Verification items for the finished model (mm, model axes). A direction names the side the tool comes from. Coordinates: 2 decimals unless noted, no trailing zeros. Order: outer loops, then holes, each group sorted by start corner. A loop starts at its lowest first (then second) coordinate and runs counter-clockwise, first axis right, second up. Notation, with made-up numbers: M 87,48.5 L 108,48.5 A20 ccw 108,83.5 Z; hole C 38.25,62.5 d7. An arc over 180 degrees is marked long. Answer as a JSON object with one key per item and string values. Group by question number.
(1) Material ranges on line 1 (Y direction, x = 5.5, z = 5); line 2 (X direction, y = 0.5, z = 5.5); line 3 (X direction, y = -7.5, z = 2.25), recorded low to high.
(2) Cross-section at B-B (y = 2.5). Enter the section's corners in (x, z), plus the area to 3 significant figures.
(3) Cross-section at D-D (y = -5.5). Enter the section's corners in (x, z).
(4) Cross-section at C-C (x = 15). Enter the section's corners in (y, z), plus the area to 3 significant figures.
(5) Gauge pin test, flat end, axial feed: pin 1 Ø1.5 at (x, y) = (-1, 1) entering from -Z. Record the tip position at first contact, or that the pin passes through.
(6) Mould release check, pull along X, two halves, no side actions. Record for faces 3 (the face through (19.05, 0, 8)), 4 (the face through (4, 4, 6)), 5 (the face through (3.9, 6.7, 4.5)), 6 (the face through (-12, 0, 0)): released by +X, released by -X, zero draft, split by the parting line, or undercut.
(7) Access from +Z, -Z, +X, -X, +Y, -Y to the whole of each face (thin tool, end or side, straight path). Record for faces 1 (the face through (4, -4, 6)), 2 (the face through (0, 0, 15.24)).
(8) Cross-section at A-A (x = 3.95). Enter the section's corners in (y, z), plus the area to 3 significant figures.
from build123d import *

# Parameters (mm, degrees)
F0_W     = 38.1
F0_H     = 13.271
F1_DEPTH = 15.24
F3_DEPTH = 8
F0_H_2   = 5.271
F4_DEPTH = 15.24
F5_R     = 4.5
F6_DEPTH = 50.8


with BuildPart() as f1:
    # F0 (on Top) → F1 (new body)
    with BuildSketch(Plane.XY):
        with Locations((0, 2.6355)):
            Rectangle(F0_W, F0_H)
    extrude(amount=F1_DEPTH)

    # F2 (on face) → F3 (cut)
    with BuildSketch(Plane.XZ.offset(4)):
        with BuildLine():
            Line((8.45, 0), (15.45, 0))
            ThreePointArc((15.45, 0), (3.95, 11.5), (-7.55, 0))
            Line((-7.55, 0), (-0.55, 0))
            ThreePointArc((-0.55, 0), (3.95, 4.5), (8.45, 0))
        make_face()
        with BuildLine():
            Line((-0.55, 0), (8.45, 0))
            ThreePointArc((8.45, 0), (3.95, 4.5), (-0.55, 0))
        make_face()
    extrude(amount=-F3_DEPTH, mode=Mode.SUBTRACT)

    # F0 (on Top) → F4 (join)
    with BuildSketch(Plane.XY):
        with Locations((0, -6.6355)):
            Rectangle(F0_W, F0_H_2)
    extrude(amount=F4_DEPTH)

    # F5 (on face) → F6 (cut)
    with BuildSketch(Plane(origin=(0, 9.271, 0), x_dir=(-1, 0, 0), z_dir=(0, 1, 0))):
        with Locations((-3.95, 0)):
            Circle(F5_R)
    extrude(amount=-F6_DEPTH, mode=Mode.SUBTRACT)


solid = f1.part
Taken from the geometry:
{
 "1": {"line 1": "y = -9.27 to -4, 4 to 9.27", "line 2": "x = -19.05 to -6.15, 14.05 to 19.05", "line 3": "x = -19.05 to 0.05, 7.85 to 19.05"},
 "2": {"outline": "M -19.05,0 L -7.55,0 A11.5 cw 15.45,0 L 19.05,0 L 19.05,15.24 L -19.05,15.24 Z", "area": "373 mm²"},
 "3": {"outline": "M -19.05,0 L -0.55,0 A4.5 cw 8.45,0 L 19.05,0 L 19.05,15.24 L -19.05,15.24 Z"},
 "4": {"outline": "M -9.27,0 L -4,0 L -4,3.19 L 4,3.19 L 4,0 L 9.27,0 L 9.27,15.24 L -9.27,15.24 Z", "area": "257 mm²"},
 "5": {"pin 1": "stops at z = 9.99"},
 "6": {"face 3": "released by +X", "face 4": "undercut", "face 5": "undercut", "face 6": "zero draft"},
 "7": {"face 1": "-Z", "face 2": "+Z, +X, -X, +Y, -Y"},
 "8": {"outline": "M -9.27,4.5 L -4,4.5 L -4,11.5 L 4,11.5 L 4,4.5 L 9.27,4.5 L 9.27,15.24 L -9.27,15.24 Z", "area": "143 mm²"}
}
